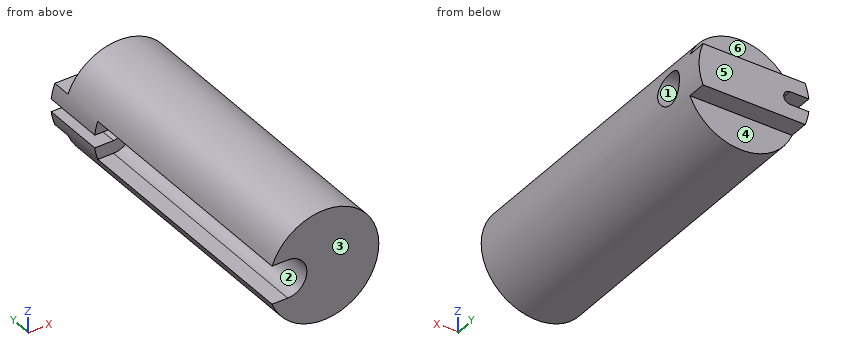
```python
from build123d import *

# Parameters (mm, degrees)
SKETCH_1_R               = 8.65
EXTRUDE_1_DEPTH          = 50
CUT_EXTRUDE_1_DEPTH      = 40
CUT_EXTRUDE_2_DEPTH      = 51
SKETCH_4_W               = 7.4
SKETCH_4_H               = 3
CUT_EXTRUDE_3_DEPTH      = 9.65
CUT_EXTRUDE_3_DEPTH_BACK = 9.592002095
HOLE_WIZARD_M61_D        = 5
HOLE_WIZARD_M61_DEPTH    = 5
HOLE_WIZARD_M61_TIP      = 1.502151548


with BuildPart() as part:
    # Эскиз1 → Бобышка-Вытянуть1 (new body)
    with BuildSketch(Plane(origin=(0, 0, 0), x_dir=(1, 0, 0), z_dir=(0, 1, 0))):
        Circle(SKETCH_1_R)
    extrude(amount=-EXTRUDE_1_DEPTH)

    # Эскиз2 → Вырез-Вытянуть1 (cut)
    with BuildSketch(Plane.XZ.offset(50)):
        with BuildLine():
            Line((-5.65, -3), (-8.65, -3))
            ThreePointArc((-8.65, -3), (-11.65, 0), (-8.65, 3))
            Line((-8.65, 3), (-5.65, 3))
            ThreePointArc((-5.65, 3), (-2.65, 0), (-5.65, -3))
        make_face()
    extrude(amount=-CUT_EXTRUDE_1_DEPTH, mode=Mode.SUBTRACT)

    # Эскиз3 → Вырез-Вытянуть2 (cut, through all)
    with BuildSketch(Plane.XZ):
        with BuildLine():
            Line((-5.65, -1), (-8.65, -1))
            ThreePointArc((-8.65, -1), (-9.65, 0), (-8.65, 1))
            Line((-8.65, 1), (-5.65, 1))
            ThreePointArc((-5.65, 1), (-4.65, 0), (-5.65, -1))
        make_face()
    extrude(amount=CUT_EXTRUDE_2_DEPTH, mode=Mode.SUBTRACT)

    # Эскиз4 → Вырез-Вытянуть3 (cut, two sides)
    with BuildSketch(Plane(origin=(0, 0, 0), x_dir=(0, 0, -1), z_dir=(1, 0, 0))) as cut_extrude_3_sk:
        with Locations((6.95, -1.5)):
            Rectangle(SKETCH_4_W, SKETCH_4_H)
        with Locations((-6.95, -1.5)):
            Rectangle(SKETCH_4_W, SKETCH_4_H)
    extrude(amount=CUT_EXTRUDE_3_DEPTH, mode=Mode.SUBTRACT)
    extrude(cut_extrude_3_sk.sketch, amount=-CUT_EXTRUDE_3_DEPTH_BACK, mode=Mode.SUBTRACT)

    # Отверстие обработанное метчиком M61
    with Locations(Plane(origin=(8.65, 0, 0), x_dir=(0, 0, -1), z_dir=(1, 0, 0))):
        with Locations((0, -7)):
            Hole(HOLE_WIZARD_M61_D / 2, depth=HOLE_WIZARD_M61_DEPTH)
            with Locations((0, 0, -(HOLE_WIZARD_M61_DEPTH + HOLE_WIZARD_M61_TIP / 2))):  # 118° drill point
                Cone(0, HOLE_WIZARD_M61_D / 2, HOLE_WIZARD_M61_TIP, mode=Mode.SUBTRACT)


solid = part.part
```
Check sheet for the modelled part. Datum: model origin and axes. Units: mm. Face numbers are marked on the shaded views. A direction names the side the tool comes from. Give positions to 0.01 mm unless a question says otherwise; leave off trailing zeros. Loops run counter-clockwise (first coordinate to the right, second up) from the corner with the lowest first, then second, coordinate; pieces in that order, holes last. Notation, with made-up numbers: (6, 19) - (28, 19) arc R30 ccw to (28, 48) - close; hole circle Ø7 at (20, 36.5). An arc over 180 degrees is marked (long way). One line per question, with ' | ' between items. Start each with the question number.
1. Material ranges on line 1 along Y through (x, z) = (4.7, 0); line 2 along Y through (x, z) = (-4.25, -1.25); line 3 along Y through (x, z) = (-3.75, 6), recorded low to high. Write a range as [from, to].
2. Cross-section at D-D, the plane z = 7. Enter the section's corners in (x, y), plus the area to 3 significant figures.
3. Set-up check for the marked faces 5 and 6: record each of +Z, -Z, +X, -X, +Y, -Y from which the full face is reachable in a straight line by a thin tool's end or side.
4. Cross-section at B-B, the plane x = 4.5. Enter the section's corners in (y, z), plus the area to 3 significant figures.
5. Cross-section at A-A, the plane x = 0. Enter the section's corners in (y, z), plus the area to 3 significant figures.
6. Gauge pin test, flat ends, axial feed: pin 1 Ø8 at (y, z) = (-7, 0) entering from -X; pin 2 Ø0.7 at (x, y) = (-6.5, -31) entering from +Z; pin 3 Ø0.9 at (x, y) = (-6.5, -3) entering from -Z; pin 4 Ø4 at (x, y) = (-3, -18.5) entering from +Z. Record the tip position at first contact, or that the pin passes through.
7. Cross-section at C-C, the plane y = -15. Enter the section's corners in (x, z), plus the area to 3 significant figures.
8. Draft check along Y on the marked faces 1, 2, 3 and 4. Enter one of: released by +Y, released by -Y, zero draft, split by the parting line, or undercut.
Check result:
1) line 1: y = [-50, -9.5], [-4.5, 0] | line 2: y = [-10, 0] | line 3: y = [-50, -3]
2) outline: (-5.08, -50) - (5.08, -50) - (5.08, -3) - (-5.08, -3) - close | area: 478 mm2
3) face 5: +Z, -Z, +X, -X, +Y | face 6: +Z, +X, -X, +Y
4) outline: (-50, -7.39) - (-3, -7.39) - (-3, -3.25) - (0, -3.25) - (0, 3.25) - (-3, 3.25) - (-3, 7.39) - (-50, 7.39) - close; hole circle Ø5 at (-7, 0) | area: 694 mm2
5) outline: (-50, -8.65) - (-3, -8.65) - (-3, -3.25) - (0, -3.25) - (0, 3.25) - (-3, 3.25) - (-3, 8.65) - (-50, 8.65) - close | area: 833 mm2
6) pin 1: stops at x = -8.59 | pin 2: stops at z = 6.08 | pin 3: stops at z = -6.18 | pin 4: stops at z = 8.59
7) outline: (-8.11, -3) arc R8.65 ccw (long way) to (-8.11, 3) - (-5.65, 3) arc R3 cw to (-5.65, -3) - close | area: 204 mm2
8) face 1: undercut | face 2: zero draft | face 3: released by -Y | face 4: released by +Y
